For this review, take the finished solid that the model builds, in its own axes (mm). A direction names the side the tool comes from. Coordinates: 2 decimals unless noted, no trailing zeros. Write each loop counter-clockwise with the first axis right and the second up, starting at its lowest first coordinate (ties: lowest second). Pieces come first, ordered by that corner, then holes.
1) Insertion check: P1, Ø10, axis at x = -13, z = 10, coming from the +Y side; P2, Ø2, axis at x = -16.5, z = -8.5, coming from the +Y side; P3, Ø8, axis at x = -18.5, y = 18.5, coming from the +Z side; P4, Ø12, axis at y = 15, z = 6.5, coming from the +X side. Each pin has a flat end and moves straight along its axis. Give the tip position at first contact, or say it passes through.
2) For faces 5 (the face through (19.243, 41, -7)), 6 (the face through (-0.623, 8.049, -4.053)), list the 3-axis set-ups (+Z, -Z, +X, -X, +Y, -Y) from which the entire face can be reached by the end or side of a thin tool; tool diameter is ignored.
3) We need section A-A on z = 0. Write out the cut boundary in (x, y) (1 decimal), then the cut area to 3 significant figures.
4) We need section C-C on z = -4. Write out the cut boundary in (x, y) (1 decimal).
5) Mouldability with a two-part tool opening along Z and no side actions: class faces 1 (the face through (11.416, 20.272, 5.168)), 2 (the face through (11.416, 22.797, -3.13)), 3 (the face through (-23.4, 0, -3.9)), 4 (the face through (-3.868, 8.049, 3.991)) as pulls with the +Z half, pulls with the -Z half, needs draft (parallel to the pull), parting line crosses it, or undercut.
6) To check wall thickness, follow line 1 along Z through (x, y) = (-9, 33.5); line 2 along Y through (x, z) = (10, -8); line 3 along Z through (x, y) = (-7, 12). State the ranges of each line that lie inside material, in increasing order.
7) We need section B-B on y = 11. Write out the cut boundary in (x, z), then the cut area to 3 significant figures.
from build123d import *

# Parameters (mm, degrees)
F1_R = 13.49375
F3_T = -3.0734


with BuildPart() as f2:
    # F2: sweep along a path in F0
    with BuildLine(Plane.XY) as f2_path:
        Line((0, 0), (0, 15.875))
        ThreePointArc((0, 15.875), (0.9863460454, 18.25625), (3.3675960454, 19.2425960454))
        Line((3.3675960454, 19.2425960454), (19.2425960454, 19.2425960454))
    # F1 (on Front) → F2 (sweep)
    with BuildSketch(Plane.XZ):
        with Locations((-13.49375, 0)):
            Circle(F1_R)
    sweep(path=f2_path.line)

    # F3
    f3_openings = [f2.faces().sort_by_distance(p)[0] for p in [
        (-13.49375, 0, 0),
        (19.242596, 32.736346, 0),
    ]]
    offset(amount=F3_T, openings=f3_openings)


solid = f2.part
Result:
1. P1: stops at y = 41.57
1. P2: stops at y = 36.12
1. P3: stops at z = 13.44
1. P4: stops at x = 19.24
2. face 5: +Z, -Z, +X, +Y, -Y
2. face 6: -Y
3. outline: (-27, 0) - (-23.9, 0) - (-23.9, 15.9) arc R27.3 cw to (3.4, 43.2) - (19.2, 43.2) - (19.2, 46.2) - (3.4, 46.2) arc R30.4 ccw to (-27, 15.9) - close; (-3.1, 0) - (0, 0) - (0, 15.9) arc R3.4 cw to (3.4, 19.2) - (19.2, 19.2) - (19.2, 22.3) - (3.4, 22.3) arc R6.4 ccw to (-3.1, 15.9) - close
3. area: 358 mm2
4. outline: (-26.4, 0) - (-23.1, 0) - (-23.1, 15.9) arc R26.5 cw to (3.4, 42.4) - (19.2, 42.4) - (19.2, 45.6) - (3.4, 45.6) arc R29.7 ccw to (-26.4, 15.9) - close; (-3.9, 0) - (-0.6, 0) - (-0.6, 15.9) arc R4 cw to (3.4, 19.8) - (19.2, 19.8) - (19.2, 23.1) - (3.4, 23.1) arc R7.2 ccw to (-3.9, 15.9) - close
5. face 1: parting line crosses it
5. face 2: undercut
5. face 3: needs draft
5. face 4: undercut
6. line 1: z = -12.66 to -9.32, 9.32 to 12.66
6. line 2: y = 21.87 to 26.06, 39.41 to 43.6
6. line 3: z = -11.83 to -8.15, 8.15 to 11.83
7. outline: circle Ø26.99 at (-13.49, 0); hole circle Ø20.84 at (-13.49, 0)
7. area: 231 mm2
